from build123d import *

# Parameters (mm, degrees)
SKETCH_1_W          = 24
SKETCH_1_H          = 31
EXTRUDE_1_DEPTH     = 5.1
SKETCH_2_W          = 24
SKETCH_2_H          = 4.1
CUT_EXTRUDE_1_DEPTH = 0.85
SKETCH_3_W          = 1.67
SKETCH_3_H          = 3
EXTRUDE_2_DEPTH     = 0.1


with BuildPart() as part:
    # Эскиз1 → Бобышка-Вытянуть1 (new body)
    with BuildSketch(Plane(origin=(0, 0, 0), x_dir=(1, 0, 0), z_dir=(0, 1, 0))):
        Rectangle(SKETCH_1_W, SKETCH_1_H)
    extrude(amount=EXTRUDE_1_DEPTH)

    # Эскиз2 → Вырез-Вытянуть1 (cut)
    with BuildSketch(Plane(origin=(0, 5.1, 0), x_dir=(1, 0, 0), z_dir=(0, 1, 0))):
        with Locations((0, 13.45)):
            Rectangle(SKETCH_2_W, SKETCH_2_H)
    extrude(amount=-CUT_EXTRUDE_1_DEPTH, mode=Mode.SUBTRACT)

    # Эскиз3 → Бобышка-Вытянуть2 (add)
    with BuildSketch(Plane(origin=(0, 4.25, 0), x_dir=(1, 0, 0), z_dir=(0, 1, 0))):
        with Locations((1.335, 13.5)):
            Rectangle(SKETCH_3_W, SKETCH_3_H)
        with Locations((3.935, 13.5)):
            Rectangle(SKETCH_3_W, SKETCH_3_H)
        with Locations((6.635, 13.5)):
            Rectangle(SKETCH_3_W, SKETCH_3_H)
    extrude(amount=EXTRUDE_2_DEPTH)


solid = part.part
Can you work these out from the model? Positions are in its coordinate system, mm. A direction names the side the tool comes from. Round coordinates to 2 decimals unless told otherwise and drop trailing zeros. Write each loop counter-clockwise with the first axis right and the second up, starting at its lowest first coordinate (ties: lowest second). Pieces come first, ordered by that corner, then holes. Notation, with made-up numbers: (4.25, 46.25) - (23.25, 46.25) arc R22 cw to (23.25, 72.25) - close; hole circle Ø7 at (-10.5, 79). An arc over 180 degrees is marked (long way). Write each question's results on one line, items separated by ' | '. Start each with the question number.
1) Which directions (+Z, -Z, +X, -X, +Y, -Y) give clear straight access to the entire face, cutting with the end or side of a thin tool? Please do faces 1 (the flat face through (0, 3, 15.5)), 2 (the flat face through (7, 4.35, -14)).
2) Suppose I cut it at B-B (z = -12.5). List the corners of the cut face in (x, y) for me, and give its area (3 significant figures).
3) Suppose I cut it at C-C (x = 3.5). List the corners of the cut face in (y, z) for me.
4) Suppose I cut it at A-A (x = -4.25). List the corners of the cut face in (y, z) for me.
5) Please list where these lines run through material, in increasing order: line 1 (Z direction, x = -3.25, y = 4.45); line 2 (Y direction, x = -0.25, z = -12).
6) For pin 1 Ø0.8 at (x, z) = (6.5, -13.5) entering from +Y, with a flat end and sliding along its axis, tell me the tip position at first contact or that it passes through.
Here are the results:
1) face 1: +Z, +X, -X, +Y, -Y | face 2: -Z, +X, -X, +Y
2) outline: (-12, 0) - (12, 0) - (12, 4.25) - (7.47, 4.25) - (7.47, 4.35) - (5.8, 4.35) - (5.8, 4.25) - (4.77, 4.25) - (4.77, 4.35) - (3.1, 4.35) - (3.1, 4.25) - (2.17, 4.25) - (2.17, 4.35) - (0.5, 4.35) - (0.5, 4.25) - (-12, 4.25) - close | area: 103 mm2
3) outline: (0, -15.5) - (4.25, -15.5) - (4.25, -15) - (4.35, -15) - (4.35, -12) - (4.25, -12) - (4.25, -11.4) - (5.1, -11.4) - (5.1, 15.5) - (0, 15.5) - close
4) outline: (0, -15.5) - (4.25, -15.5) - (4.25, -11.4) - (5.1, -11.4) - (5.1, 15.5) - (0, 15.5) - close
5) line 1: z = -11.4 to 15.5 | line 2: y = 0 to 4.25
6) pin 1: stops at y = 4.35
